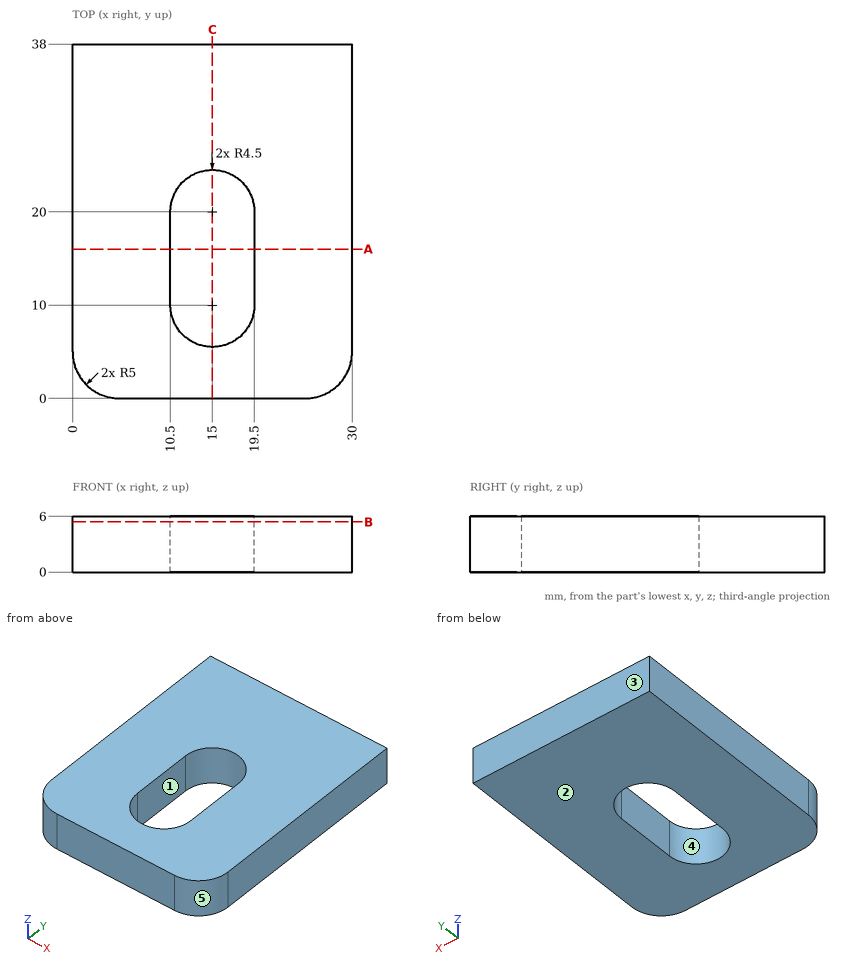
Here's the drawing with two shaded views (mm, measured from the low corner). I have some questions. A direction names the side the tool comes from. Coordinates: 2 decimals unless noted, no trailing zeros. Loops run counter-clockwise (first coordinate to the right, second up) from the corner with the lowest first, then second, coordinate; pieces in that order, holes last. Notation, with made-up numbers: (-4, -8.75) - (26, -8.75) arc R13 cw to (26, 4.25) - close; hole circle Ø10 at (-11.75, 80.25). An arc over 180 degrees is marked (long way). Answer as CSV lines item,"result". Start each with the question number.
1) Suppose I cut it at A-A (y = 16). Please give me the cut outline in (x, z).
2) Suppose I cut it at C-C (x = 15). Please give me the cut outline in (y, z), plus the area to 3 significant figures.
3) Suppose I cut it at B-B (z = 5.4). Please give me the cut outline in (x, y), plus the area to 3 significant figures.
4) I need wall thicknesses on line 1 (X direction, y = 18, z = 4.65); line 2 (Y direction, x = 14.5, z = 3.8); line 3 (Y direction, x = 25.25, z = 4.4). Which ranges of each line are inside material? Lowest first, please. Write a range as from..to.
5) Thinking about a two-plate mould opening in Y: for the marked faces 3, 4 and 5, which applies, pulls with the +Y half, pulls with the -Y half, needs draft (parallel to the pull), parting line crosses it, or undercut?
6) Which directions (+Z, -Z, +X, -X, +Y, -Y) give clear straight access to the entire face, cutting with the end or side of a thin tool? Please do the marked faces 1 and 2.
Check result:
1,outline,"(0, 0) - (10.5, 0) - (10.5, 6) - (0, 6) - close; (19.5, 0) - (30, 0) - (30, 6) - (19.5, 6) - close"
2,outline,"(0, 0) - (5.5, 0) - (5.5, 6) - (0, 6) - close; (24.5, 0) - (38, 0) - (38, 6) - (24.5, 6) - close"
2,area,"114 mm²"
3,outline,"(0, 5) arc R5 ccw to (5, 0) - (25, 0) arc R5 ccw to (30, 5) - (30, 38) - (0, 38) - close; hole (10.5, 10) arc R4.5 ccw to (19.5, 10) - (19.5, 20) arc R4.5 ccw to (10.5, 20) - close"
3,area,"976 mm²"
4,line 1,"x = 0..10.5, 19.5..30"
4,line 2,"y = 0..5.53, 24.47..38"
4,line 3,"y = 0.01..38"
5,face 3,"pulls with the +Y half"
5,face 4,"undercut"
5,face 5,"pulls with the -Y half"
6,face 1,"+Z, -Z"
6,face 2,"-Z, +X, -X, +Y, -Y"
